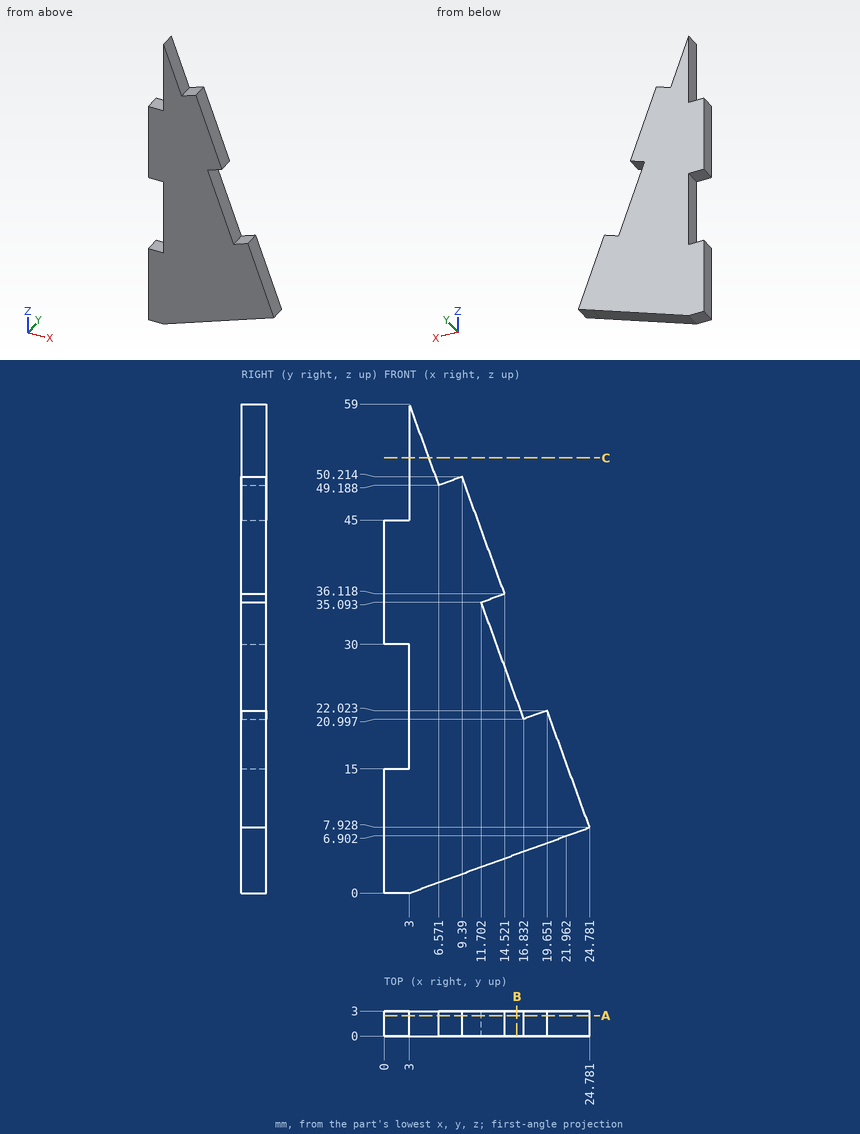
The drawing under review shows one solid part. Ordinate dimensions are in mm from its lowest x, y, z. Give positions to 0.01 mm unless a question says otherwise; leave off trailing zeros. Loops run counter-clockwise (first coordinate to the right, second up) from the corner with the lowest first, then second, coordinate; pieces in that order, holes last. Notation, with made-up numbers: M 89,-26.5 L 124,-26.5 A22 ccw 124,3.5 Z; hole C -33,44.5 d2. An arc over 180 degrees is marked long. Return JSON: item names as keys, results as strings. Group by question number.
Item 1: We need section A-A (y = 2.45). Give the boundary of the cut face in (x, z).
Item 2: For probe 1 along Z at (x, y) = (1.5, 0.2); probe 2 along X at (y, z) = (1.8, 26); probe 3 along X at (y, z) = (2.6, 15.5) (1 decimal), list the stretches that pass through material, from the lowest coordinate up.
Item 3: Insertion check: pin 1 Ø1 at (x, y) = (20.5, 1) entering from -Z; pin 2 Ø1 at (x, y) = (13.5, 2.5) entering from -Z; pin 3 Ø1.5 at (x, y) = (2, 1.5) entering from +Z. Each pin has a flat end and moves straight along its axis. Give the tip position at first contact, or say it passes through.
Item 4: We need section B-B (x = 16). Give the boundary of the cut face in (y, z).
Item 5: We need section C-C (z = 52.5). Give the boundary of the cut face in (x, y) (1 decimal).
Output:
{
 "1": {"outline": "M 0,0 L 3,0 L 21.96,6.9 L 24.78,7.93 L 19.65,22.02 L 16.83,21 L 11.7,35.09 L 14.52,36.12 L 9.39,50.21 L 6.57,49.19 L 3,59 L 3,45 L 0,45 L 0,30 L 3,30 L 3,15 L 0,15 Z"},
 "2": {"probe 1": "z = 0 to 15, 30 to 45", "probe 2": "x = 3 to 15.01", "probe 3": "x = 3 to 22"},
 "3": {"pin 1": "stops at z = 6.19", "pin 2": "stops at z = 3.64", "pin 3": "stops at z = 45"},
 "4": {"outline": "M 0,4.73 L 3,4.73 L 3,23.28 L 0,23.28 Z"},
 "5": {"outline": "M 3,0 L 5.4,0 L 5.4,3 L 3,3 Z"}
}
